Source: CAD feature listing. Evaluate the final solid. Frame: model axes, mm. Face numbers are marked on the shaded views. Give positions to 0.01 mm unless a question says otherwise; leave off trailing zeros. Loops run counter-clockwise (first coordinate to the right, second up) from the corner with the lowest first, then second, coordinate; pieces in that order, holes last. Notation, with made-up numbers: M 69,14.5 L 82,14.5 A16 ccw 82,35.5 Z; hole C -25.75,68.5 d6. An arc over 180 degrees is marked long. Put each result on its own line as item: value.
from build123d import *

# Parameters (mm, degrees)
BOSS_EXTRUDE1_DEPTH = 15
SKETCH2_R           = 1
CUT_EXTRUDE1_DEPTH  = 5
SKETCH3_W           = 16
SKETCH3_H           = 9
SKETCH3_W_2         = 15
SKETCH3_H_2         = 8
BOSS_EXTRUDE2_DEPTH = 5
SKETCH4_R           = 1
CUT_EXTRUDE2_DEPTH  = 5


with BuildPart() as part:
    # Sketch1 → Boss-Extrude1 (new body)
    with BuildSketch(Plane.XY):
        with BuildLine():
            Line((0, 0), (90, 0))
            Line((90, 0), (90, -20))
            Line((90, -20), (80, -20))
            ThreePointArc((80, -20), (45, -14.782402832), (10, -20))
            Line((10, -20), (0, -20))
            Line((0, -20), (0, 0))
        make_face()
    extrude(amount=BOSS_EXTRUDE1_DEPTH)

    # Sketch2 → Cut-Extrude1 (cut)
    with BuildSketch(Plane.XY.offset(15)):
        with Locations((7, -16)):
            Circle(SKETCH2_R)
        with Locations((83, -16)):
            Circle(SKETCH2_R)
    extrude(amount=-CUT_EXTRUDE1_DEPTH, mode=Mode.SUBTRACT)

    # Sketch3 → Boss-Extrude2 (add)
    with BuildSketch(Plane(origin=(0, 0, 0), x_dir=(-1, 0, 0), z_dir=(0, 0, -1))):
        with Locations((-45, -7)):
            Rectangle(SKETCH3_W, SKETCH3_H)
        with Locations((-45, -7)):
            Rectangle(SKETCH3_W_2, SKETCH3_H_2, mode=Mode.SUBTRACT)
    extrude(amount=BOSS_EXTRUDE2_DEPTH)

    # Sketch4 → Cut-Extrude2 (cut)
    with BuildSketch(Plane(origin=(0, 0, 0), x_dir=(-1, 0, 0), z_dir=(0, 0, -1))):
        with Locations((-45, -7)):
            Circle(SKETCH4_R)
    extrude(amount=-CUT_EXTRUDE2_DEPTH, mode=Mode.SUBTRACT)


solid = part.part
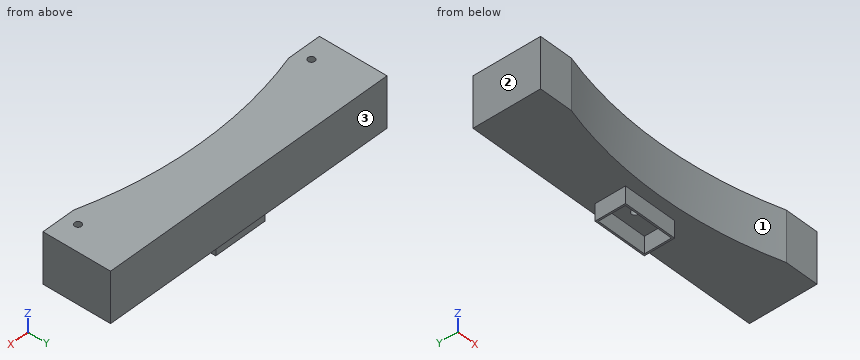
1. Contact query for flat-ended pins moving along their axis: P1, Ø1.5, axis at x = 16.5, y = -7.5, coming from the -Z side; P2, Ø0.6, axis at x = 7, y = -16.5, coming from the +Z side; P3, Ø8, axis at x = 53, z = 6, coming from the -Y side. Output: stop coordinate, or through.
Found:
P1: z = 0
P2: z = 10
P3: y = -15.38
2. Material intervals for line 1 (Y direction, x = 83, z = 12.6); line 2 (Y direction, x = 51, z = -2.5); line 3 (Z direction, x = 45, y = -3.25), sorted ascending. Write a range as from..to.
Found:
line 1: -20..-17, -15..0
line 2: -11.5..-11, -3..-2.5
line 3: 0..15
3. Section query A-A (z = -2.5). Output: boundary loops of the cut face in (x, y).
Found:
outline: M 37,-11.5 L 53,-11.5 L 53,-2.5 L 37,-2.5 Z; hole M 37.5,-11 L 52.5,-11 L 52.5,-3 L 37.5,-3 Z
4. Section query D-D (y = -7). Output: boundary loops of the cut face in (x, z).
Found:
outline: M 0,0 L 37,0 L 37,-5 L 37.5,-5 L 37.5,0 L 44,0 L 44,5 L 46,5 L 46,0 L 52.5,0 L 52.5,-5 L 53,-5 L 53,0 L 90,0 L 90,15 L 0,15 Z
5. Section query B-B (y = -16). Output: boundary loops of the cut face in (x, z), plus the area to 3 significant figures.
Found:
outline: M 0,0 L 27.95,0 L 27.95,15 L 8,15 L 8,10 L 6,10 L 6,15 L 0,15 Z; M 62.05,0 L 90,0 L 90,15 L 84,15 L 84,10 L 82,10 L 82,15 L 62.05,15 Z
area: 818 mm^2
6. Section query C-C (x = 45). Output: boundary loops of the cut face in (y, z).
Found:
outline: M -14.78,0 L -11.5,0 L -11.5,-5 L -11,-5 L -11,0 L -8,0 L -8,5 L -6,5 L -6,0 L -3,0 L -3,-5 L -2.5,-5 L -2.5,0 L 0,0 L 0,15 L -14.78,15 Z
7. Draft query along X for the marked faces 1, 2 and 3. Return one class per face: pulls with the +X half, pulls with the -X half, needs draft (parallel to the pull), parting line crosses it, or undercut.
Found:
face 1: undercut
face 2: pulls with the -X half
face 3: needs draft
